The drawing under review shows one solid part. Ordinate dimensions are in mm from its lowest x, y, z. A direction names the side the tool comes from. Give positions to 0.01 mm unless a question says otherwise; leave off trailing zeros. Order: outer loops, then holes, each group sorted by start corner. A loop starts at its lowest first (then second) coordinate and runs counter-clockwise, first axis right, second up. Notation, with made-up numbers: (60, 79) - (87, 79) arc R15 ccw to (87, 83) - close; hole circle Ø4 at (-29.5, -35.5). An arc over 180 degrees is marked (long way). Write item = value, one per line. Start each with the question number.
1. Mouldability with a two-part tool opening along X and no side actions: class the marked faces 1, 2 and 3 as pulls with the +X half, pulls with the -X half, needs draft (parallel to the pull), parting line crosses it, or undercut.
2. Machinability: for the marked faces 4 and 5, which of the approach directions +Z, -Z, +X, -X, +Y, -Y give a long, thin tool a straight path to every point of the face, cutting with its end or side? Answer none if there is none.
3. Wall thickness on probe 1 along X at (y, z) = (5.5, 13.25); probe 2 along X at (y, z) = (5.5, 16.5); probe 3 along Z at (x, y) = (4, 2.5): over which ranges is each line inside the solid? List them lowest first.
4. We need section A-A, the plane z = 13.25. Give the boundary of the cut face in (x, y).
5. For P1, Ø5, axis at y = 6, z = 14, coming from the +X side; P2, Ø4, axis at x = 18.5, z = 2.5, coming from the -Y side; P3, Ø2.5, axis at y = 4.5, z = 11.5, coming from the +X side; P4, Ø5, axis at x = 48.5, y = 6, coming from the +Z side, all flat-tipped, find the tip position at first contact; note any pin that passes through.
6. We need section C-C, the plane y = 8. Give the boundary of the cut face in (x, z).
7. We need section D-D, the plane z = 22. Give the boundary of the cut face in (x, y).
8. We need section B-B, the plane y = 2.5. Give the boundary of the cut face in (x, z), and give its area (4 significant figures).
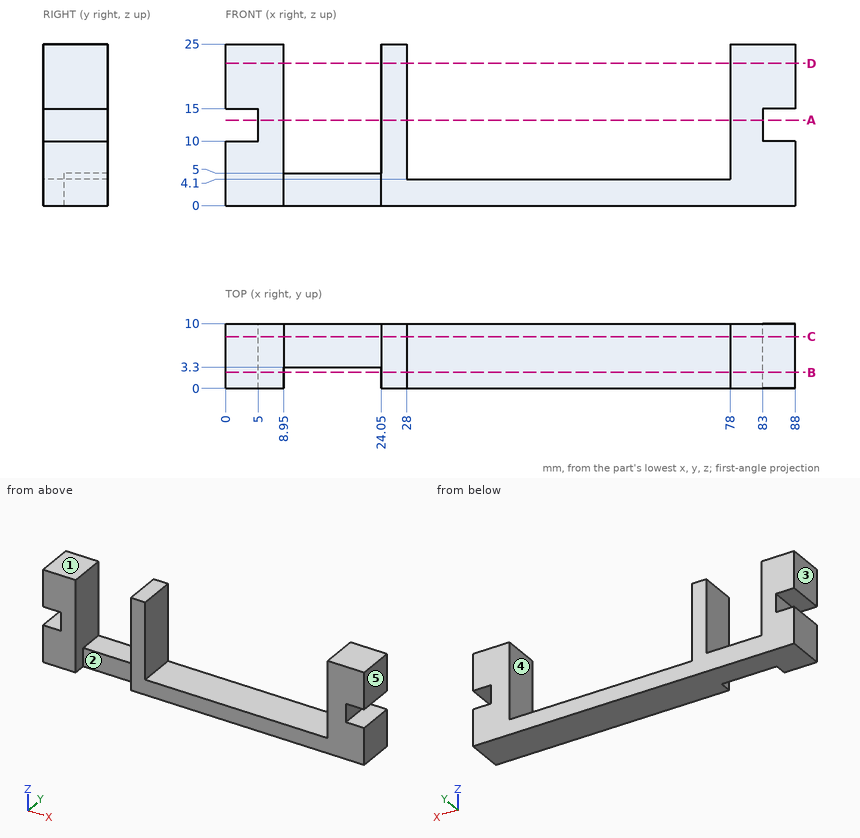
Model answer:
q1.face_1 = needs draft
q1.face_2 = undercut
q1.face_3 = pulls with the -X half
q2.face_4 = +Z, +Y, -Y
q2.face_5 = +Z, -Z, +X, +Y, -Y
q3.probe_1 = 5 to 8.95, 24.05 to 28, 78 to 83
q3.probe_2 = 0 to 8.95, 24.05 to 28, 78 to 88
q3.probe_3 = 0 to 10, 15 to 25
q4.outline = (5, 0) - (8.95, 0) - (8.95, 10) - (5, 10) - close; (24.05, 0) - (28, 0) - (28, 10) - (24.05, 10) - close; (78, 0) - (83, 0) - (83, 10) - (78, 10) - close
q5.P1 = 88
q5.P2 = 3.3
q5.P3 = 83
q5.P4 = 4.1
q6.outline = (0, 0) - (88, 0) - (88, 10) - (83, 10) - (83, 15) - (88, 15) - (88, 25) - (78, 25) - (78, 4.1) - (28, 4.1) - (28, 25) - (24.05, 25) - (24.05, 5) - (8.95, 5) - (8.95, 25) - (0, 25) - (0, 15) - (5, 15) - (5, 10) - (0, 10) - close
q7.outline = (0, 0) - (8.95, 0) - (8.95, 10) - (0, 10) - close; (24.05, 0) - (28, 0) - (28, 10) - (24.05, 10) - close; (78, 0) - (88, 0) - (88, 10) - (78, 10) - close
q8.outline = (0, 0) - (8.95, 0) - (8.95, 25) - (0, 25) - (0, 15) - (5, 15) - (5, 10) - (0, 10) - close; (24.05, 0) - (88, 0) - (88, 10) - (83, 10) - (83, 15) - (88, 15) - (88, 25) - (78, 25) - (78, 4.1) - (28, 4.1) - (28, 25) - (24.05, 25) - close
q8.area = 727.5 mm2
